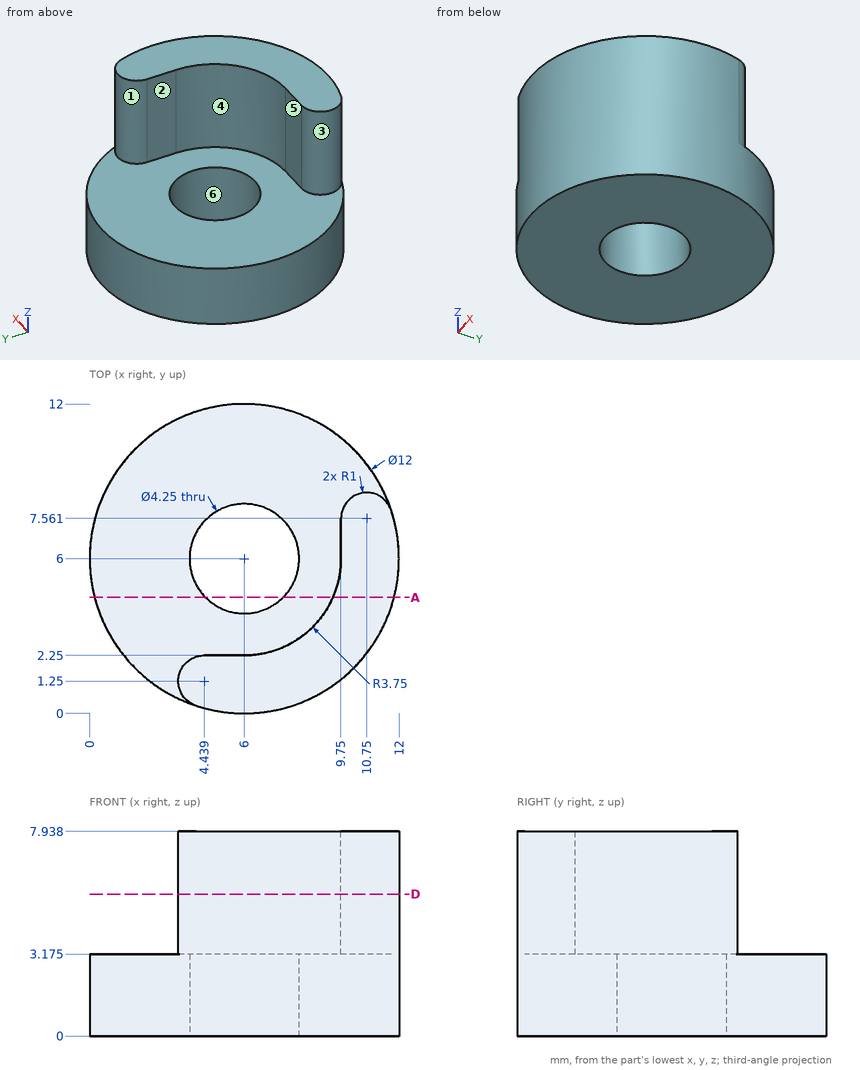
Could you check a few things on this drawing? It's one solid part, dimensions in mm from its lowest x, y, z. A direction names the side the tool comes from. Coordinates: 2 decimals unless noted, no trailing zeros. Order: outer loops, then holes, each group sorted by start corner. A loop starts at its lowest first (then second) coordinate and runs counter-clockwise, first axis right, second up. Notation, with made-up numbers: (67, 13) - (86, 13) arc R22 ccw to (86, 29) - close; hole circle Ø4 at (19, -10.5). An arc over 180 degrees is marked (long way). One line per question, with ' | ' between items. Start each with the question number.
1. Please list where these lines run through material, in increasing order: line 1 along Y through (x, z) = (6, 0.9) (1 decimal); line 2 along Z through (x, y) = (7.75, 4.75) (1 decimal); line 3 along X through (y, z) = (4.5, 1) (1 decimal). Write a range as [from, to].
2. If we mould it in two halves opening along X, with no side actions, what happens to the marked faces 4, 5 and 6? For each: released by +X, released by -X, zero draft, split by the parting line, or undercut.
3. If we section it at D-D (z = 5.5): Write out the boundary of the cut face in (x, y).
4. If we section it at A-A (y = 4.5): Write out the boundary of the cut face in (x, z) (1 decimal).
5. Which directions (+Z, -Z, +X, -X, +Y, -Y) give clear straight access to the entire face, cutting with the end or side of a thin tool? Please do the marked faces 1, 2 and 3.
6. I'm going to push flat-ended pins straight in: pin 1 Ø3 at (y, z) = (9, 6.5) entering from -X; pin 2 Ø0.5 at (x, z) = (5, 5.5) entering from +Y; pin 3 Ø3.5 at (x, y) = (6, 7) entering from +Z (1 decimal). Where does each tip first touch, or does it pass through?
Model answer:
1) line 1: y = [0, 3.9], [8.1, 12] | line 2: z = [0, 3.2] | line 3: x = [0.2, 4.5], [7.5, 11.8]
2) face 4: released by -X | face 5: zero draft | face 6: undercut
3) outline: (4.13, 0.3) arc R6 ccw to (11.7, 7.87) arc R1 ccw to (9.75, 7.56) - (9.75, 6) arc R3.75 cw to (6, 2.25) - (4.44, 2.25) arc R1 ccw to start
4) outline: (0.2, 0) - (4.5, 0) - (4.5, 3.2) - (0.2, 3.2) - close; (7.5, 0) - (11.8, 0) - (11.8, 7.9) - (9.4, 7.9) - (9.4, 3.2) - (7.5, 3.2) - close
5) face 1: +Z, +Y | face 2: +Z, -X, +Y | face 3: +Z, -X
6) pin 1: stops at x = 9.75 | pin 2: stops at y = 2.25 | pin 3: stops at z = 3.2
